```python
from build123d import *

# Parameters (mm, degrees)
BOSS_EXTRUDE1_DEPTH   = 200
BOSS_EXTRUDE1_2_DEPTH = 200
FILLET1_R             = 0.5
FILLET2_R             = 0.5
BOSS_EXTRUDE3_DEPTH   = 200
FILLET3_R             = 10
FILLET4_R             = 1
FILLET5_R             = 3
CUT_EXTRUDE2_DEPTH    = 20
CUT_EXTRUDE4_DEPTH    = 10


with BuildPart() as part:
    # Sketch1 → Boss-Extrude1 (new body)
    with BuildSketch(Plane(origin=(0, 0, 0), x_dir=(1, 0, 0), z_dir=(0, 1, 0))):
        Polygon((13.927082127, 14.175350351), (16.351953258, 13.843299543), (16.851953258, 12.977274139), (3.059579159, 5.014243241), (2.594699496, 5.900545381), (13.927082127, 12.443299543), align=None)
    extrude(amount=BOSS_EXTRUDE1_DEPTH)

    # Fillet2
    fillet2_edges = [part.edges().sort_by_distance(p)[0] for p in [
        (13.927082127, 100, -14.175350351),
        (16.351953258, 100, -13.843299543),
        (13.927082127, 100, -12.443299543),
    ]]
    fillet(fillet2_edges, radius=FILLET2_R)



with BuildPart() as body_2:
    # Sketch1 → Boss-Extrude1 2 (new body)
    with BuildSketch(Plane(origin=(0, 0, 0), x_dir=(1, 0, 0), z_dir=(0, 1, 0))):
        Polygon((18.751953258, 9.686377605), (19.251953258, 8.820352201), (18.153877046, 6.454326797), (16.653877046, 7.320352201), (5.114206816, 0.657920487), (4.719127398, 1.584521817), align=None)
    extrude(amount=BOSS_EXTRUDE1_2_DEPTH)

    # Fillet1
    fillet1_edges = [body_2.edges().sort_by_distance(p)[0] for p in [
        (19.251953258, 100, -8.820352201),
        (18.153877046, 100, -6.454326797),
        (16.653877046, 100, -7.320352201),
    ]]
    fillet(fillet1_edges, radius=FILLET1_R)


with BuildPart() as part_1:
    add(part.part)

    add(body_2.part)  # Boss-Extrude3 merges body 2
    # Sketch2 → Boss-Extrude3 (add)
    with BuildSketch(Plane(origin=(0, 0, 0), x_dir=(1, 0, 0), z_dir=(0, 1, 0))):
        Polygon((8.182648293, 2.429486), (3.232648293, 11.003137498), (10.393111947, 15.137233116), (8.893111947, 17.735309327), (1.732648293, 13.601213709), (-13.163737181, -4.647533202), (-9.075108531, -18.787281313), (-9.075108531, -4.647533202), (-4.075108531, -4.647533202), align=None)
    extrude(amount=BOSS_EXTRUDE3_DEPTH)

    # Fillet3
    fillet3_edges = [part_1.edges().sort_by_distance(p)[0] for p in [
        (-13.163737181, 100, 4.647533202),
    ]]
    fillet(fillet3_edges, radius=FILLET3_R)

    # Fillet4
    fillet4_edges = [part_1.edges().sort_by_distance(p)[0] for p in [
        (5.782648293, 100, -6.586407938),
        (7.682648293, 100, -3.295511404),
    ]]
    fillet(fillet4_edges, radius=FILLET4_R)

    # Fillet5
    fillet5_edges = [part_1.edges().sort_by_distance(p)[0] for p in [
        (3.232648293, 100, -11.003137498),
    ]]
    fillet(fillet5_edges, radius=FILLET5_R)

    # Sketch3 → Cut-Extrude2 (cut)
    with BuildSketch(Plane(origin=(0, 0, 0), x_dir=(1, 0, 0), z_dir=(0, 1, 0))):
        with BuildLine():
            Line((-6.589903921, 8.016296992), (-2.313602471, 0.609525612))
            ThreePointArc((-2.313602471, 0.609525612), (-4.361026605, -1.438580666), (-1.563602471, -0.689512493))
            Line((-1.563602471, -0.689512493), (0.970355299, -5.078456095))
            Line((0.970355299, -5.078456095), (0.623945137, -5.278456095))
            Line((0.623945137, -5.278456095), (-1.448316815, -1.689193106))
            ThreePointArc((-1.448316815, -1.689193106), (-4.707436766, -1.638580666), (-3.12170845, 1.209206225))
            Line((-3.12170845, 1.209206225), (-6.936314083, 7.816296992))
            Line((-6.936314083, 7.816296992), (-6.589903921, 8.016296992))
        make_face()
    extrude(amount=CUT_EXTRUDE2_DEPTH, mode=Mode.SUBTRACT)

    # Sketch4 → Cut-Extrude4 (cut)
    with BuildSketch(Plane(origin=(0, 0, 0), x_dir=(1, 0, 0), z_dir=(0, 1, 0))):
        with BuildLine():
            Line((-2.313602471, 0.609525612), (-5.030743669, 5.315752219))
            Line((-5.030743669, 5.315752219), (-2.055391297, 8.960693639))
            Line((-2.055391297, 8.960693639), (4.693297418, 0.414908333))
            Line((4.693297418, 0.414908333), (-0.477605745, -2.570514))
            Line((-0.477605745, -2.570514), (-1.563602471, -0.689512493))
            ThreePointArc((-1.563602471, -0.689512493), (-1.76444841, 0.060554453), (-2.313602471, 0.609525612))
        make_face()
    extrude(amount=CUT_EXTRUDE4_DEPTH, mode=Mode.SUBTRACT)


solid = part_1.part
```
Build history of the part. All positions in model axes, mm. A direction names the side the tool comes from. Coordinates: 2 decimals unless noted, no trailing zeros. Order: outer loops, then holes, each group sorted by start corner. A loop starts at its lowest first (then second) coordinate and runs counter-clockwise, first axis right, second up. Notation, with made-up numbers: (30.25, -9.5) -> (75.25, -9.5) arc R29 cw to (75.25, 22.5) -> close; hole circle Ø2 at (16, 5). An arc over 180 degrees is marked (long way). Answer in a Markdown table with one row per item. Add a question column.
Q1. Which spindle directions (+Z, -Z, +X, -X, +Y, -Y) get a long thin tool onto all of the face, cutting with end or side? Do faces 5 (the face through (1.27, 4.93, -4.75)), 6 (the face through (11.82, 98.6, -10.07)), 7 (the face through (-8, 0, 4)). Say none if no direction does.
Q2. Band-saw the part on B-B, the plane z = 6.5. List the corners of the cut face in (x, y), then the cut area to 3 significant figures.
Q3. Mould opens along X. For faces 1 (the face through (-10.4, 98.6, 14.2)), 2 (the face through (0, 200, -4)), 3 (the face through (-9.075, 99, 12)), 4 (the face through (-4.196, 9.86, -3.07)) say: +X half, -X half, draft (parallel to the pull), parting line (faces both ways), or undercut.
Q4. Drop flat-ended pins along their axis: pin 1 (5.5 mm diameter, centred on x = -5.5, y = 137, fed in from +Z); pin 2 (1 mm diameter, centred on x = 15, z = -9.5, fed in from +Y); pin 3 (4 mm diameter, centred on x = 8.5, z = -2.5, fed in from -Y); pin 4 (2 mm diameter, centred on y = 52, z = 5.5, fed in from +X). Give the stop position or say it passes through.
Q5. Wall check: line 1 along X through (y, z) = (39.5, -9.5); line 2 along X through (y, z) = (82.5, 6.5); line 3 along Z through (x, y) = (10, 148.5). Give the ranges that are in metal, low to high. Write a range as [from, to].
Answers follow:
| question | item | result |
|---|---|---|
| 1 | face 5 | -Y |
| 1 | face 6 | +Y, -Y |
| 1 | face 7 | +Z, -Z, +X, -X, -Y |
| 2 | outline | (-12.09, 0) -> (-9.08, 0) -> (-9.08, 200) -> (-12.09, 200) -> close |
| 2 | area | 603 mm^2 |
| 3 | face 1 | -X half |
| 3 | face 2 | draft |
| 3 | face 3 | +X half |
| 3 | face 4 | undercut |
| 4 | pin 1 | z = 4.65 |
| 4 | pin 2 | through |
| 4 | pin 3 | y = 0 |
| 4 | pin 4 | x = -3.82 |
| 5 | line 1 | [-1.62, 4.36], [8.83, 10.83], [18.43, 18.86] |
| 5 | line 2 | [-12.09, -9.08] |
| 5 | line 3 | [-15.82, -14.91], [-10.18, -9.02], [-4.63, -3.48] |
